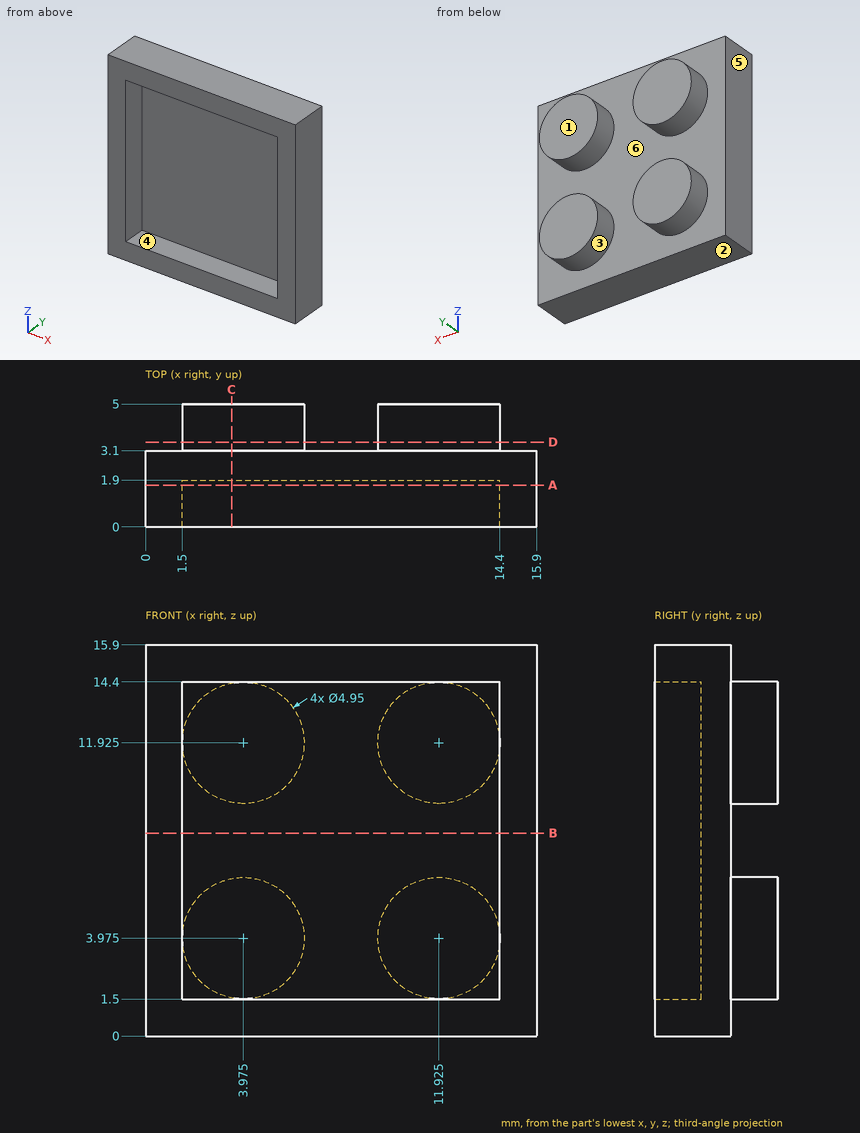
Answer from the drawing. Dimensions are ordinates in mm from the lowest x, y and z of the part. A direction names the side the tool comes from. Coordinates: 2 decimals unless noted, no trailing zeros. Write each loop counter-clockwise with the first axis right and the second up, starting at its lowest first coordinate (ties: lowest second). Pieces come first, ordered by that corner, then holes. Notation, with made-up numbers: M 51,45 L 91,45 A23 cw 91,53 Z; hole C 74,80.25 d3. An arc over 180 degrees is marked long. Use one line per item in the form item = value. Start each with the question number.
1. The part is cut by section D-D (y = 3.45). Give the vertices of the cut face in (x, z) (3 decimals).
2. The part is cut by section A-A (y = 1.7). Give the vertices of the cut face in (x, z).
3. Each of these flat-tipped pins is pushed along its axis until it touches: P1, Ø6.5, axis at x = 8, z = 9, coming from the -Y side; P2, Ø1, axis at x = 2.5, z = 8, coming from the +Y side. Where does it stop, or does it pass through?
4. Straight lines are drawn through the part: probe 1 along X at (y, z) = (1.75, 10.5); probe 2 along Y at (x, z) = (9.25, 1.75). For each, find the intervals that lie inside material, in ascending order. Write a range as from..to.
5. The mould has two halves that part along Z. Classify the marked faces 1, 2 and 3: released by +Z, released by -Z, zero draft, split by the parting line, or undercut.
6. The part is cut by section B-B (z = 8.25). Give the vertices of the cut face in (x, y), plus the area to 3 significant figures.
7. A tool of negligible diameter and unlimited length cuts with its end or side. For the marked faces 4, 5 and 6, from which of +Z, -Z, +X, -X, +Y, -Y can it reach the whole face along a straight path? Write none if from no direction.
8. The part is cut by section C-C (x = 3.5). Give the vertices of the cut face in (y, z).
Evaluation:
q1.outline = C 3.975,3.975 d4.95; C 3.975,11.925 d4.95; C 11.925,3.975 d4.95; C 11.925,11.925 d4.95
q2.outline = M 0,0 L 15.9,0 L 15.9,15.9 L 0,15.9 Z; hole M 1.5,1.5 L 14.4,1.5 L 14.4,14.4 L 1.5,14.4 Z
q3.P1 = 1.9
q3.P2 = 3.1
q4.probe_1 = 0..1.5, 14.4..15.9
q4.probe_2 = 1.9..3.1
q5.face_1 = zero draft
q5.face_2 = released by -Z
q5.face_3 = undercut
q6.outline = M 0,0 L 1.5,0 L 1.5,1.9 L 14.4,1.9 L 14.4,0 L 15.9,0 L 15.9,3.1 L 0,3.1 Z
q6.area = 24.8 mm^2
q7.face_4 = -Y
q7.face_5 = +Z, -Z, -X, +Y, -Y
q7.face_6 = +Y
q8.outline = M 0,0 L 3.1,0 L 3.1,1.55 L 5,1.55 L 5,6.4 L 3.1,6.4 L 3.1,9.5 L 5,9.5 L 5,14.35 L 3.1,14.35 L 3.1,15.9 L 0,15.9 L 0,14.4 L 1.9,14.4 L 1.9,1.5 L 0,1.5 Z
